```python
from build123d import *

# Parameters (mm, degrees)
BOSS_EXTRUDE1_DEPTH = 31
SKETCH4_W           = 25
SKETCH4_H           = 15
CUT_EXTRUDE2_DEPTH  = 25
CUT_EXTRUDE4_DEPTH  = 11.5
SKETCH7_W           = 31
SKETCH7_H           = 1.7
BOSS_EXTRUDE3_DEPTH = 7
BOSS_EXTRUDE4_DEPTH = 7
LPATTERN1_COUNT     = 8
LPATTERN1_PITCH     = 4
SKETCH11_W          = 12
SKETCH11_H          = 6.5
BOSS_EXTRUDE5_DEPTH = 5.5
FILLET5_R           = 3
SKETCH12_W          = 12
SKETCH12_H          = 6.5
BOSS_EXTRUDE6_DEPTH = 6
CUT_EXTRUDE5_DEPTH  = 12
FILLET6_R           = 2


with BuildPart() as part:
    # Sketch1 → Boss-Extrude1 (new body)
    with BuildSketch(Plane.XY):
        Polygon((0, 0), (0, -30), (12, -30), (12, -20), (5, 0), align=None)
    extrude(amount=-BOSS_EXTRUDE1_DEPTH)

    # Sketch4 → Cut-Extrude2 (cut)
    with BuildSketch(Plane.ZY):
        with Locations((-15, -24.143402944)):
            Rectangle(SKETCH4_W, SKETCH4_H)
    extrude(amount=-CUT_EXTRUDE2_DEPTH, mode=Mode.SUBTRACT)

    # Sketch6 → Cut-Extrude4 (cut, symmetric)
    with BuildSketch(Plane.XY.offset(-15.25)):
        Polygon((5, 0), (5, -14), (9.9, -14), align=None)
    extrude(amount=CUT_EXTRUDE4_DEPTH, both=True, mode=Mode.SUBTRACT)

    # Sketch7 → Boss-Extrude3 (add)
    with BuildSketch(Plane(origin=(0, -25.5, 0), x_dir=(1, 0, 0), z_dir=(0, 1, 0))):
        with Locations((-4.2231607, 26.8)):
            Rectangle(SKETCH7_W, SKETCH7_H)
    extrude(amount=BOSS_EXTRUDE3_DEPTH)

    # Sketch10 → Boss-Extrude4 (add)
    with BuildSketch(Plane(origin=(0, -25.5, 0), x_dir=(1, 0, 0), z_dir=(0, 1, 0))):
        with BuildLine():
            Line((10.353586314, 22.126900466), (9.550714712, 22.126900466))
            ThreePointArc((9.550714712, 22.126900466), (8.911730102, 23.551984668), (9.029666421, 25.109308443))
            ThreePointArc((9.029666421, 25.109308443), (8.752067329, 25.53731984), (8.452150513, 25.95))
            Line((8.452150513, 25.95), (11.452150513, 25.95))
            ThreePointArc((11.452150513, 25.95), (11.152233697, 25.53731984), (10.874634605, 25.109308443))
            ThreePointArc((10.874634605, 25.109308443), (10.992570924, 23.551984668), (10.353586314, 22.126900466))
        make_face()
    boss_extrude4 = extrude(amount=BOSS_EXTRUDE4_DEPTH)

    # LPattern1: Boss-Extrude4 ×8
    with Locations(*[(-i * LPATTERN1_PITCH, 0, 0) for i in range(1, LPATTERN1_COUNT)]):
        add(boss_extrude4)

    # Sketch11 → Boss-Extrude5 (add)
    with BuildSketch(Plane(origin=(0, 0, -31), x_dir=(-1, 0, 0), z_dir=(0, 0, -1))):
        with Locations((-6, -26.75)):
            Rectangle(SKETCH11_W, SKETCH11_H)
    extrude(amount=BOSS_EXTRUDE5_DEPTH)

    # Fillet5
    # the kernel refuses this fillet: 3 mm, written as the material it adds along each edge
    with BuildSketch(Plane(origin=(5, -14, -34.25), x_dir=(0, 1, 0), z_dir=(0, 0, 1))) as fillet5_piece_1_section:
        with BuildLine():
            CenterArc((FILLET5_R, -FILLET5_R), FILLET5_R, 90, 90)
            Line((0, -FILLET5_R), (0, 0))
            Line((0, 0), (FILLET5_R, 0))
        make_face()
    fillet5_piece_1 = extrude(amount=38, mode=Mode.PRIVATE)
    fillet5_piece_1 = split(fillet5_piece_1, bisect_by=Plane(origin=(5.670103817, -13.329896183, -31), z_dir=(0, 0, 1)), keep=Keep.TOP, mode=Mode.PRIVATE)
    fillet5_piece_1 = split(fillet5_piece_1, bisect_by=Plane(origin=(5.670103817, -13.329896183, 0), z_dir=(0, 0, -1)), keep=Keep.TOP, mode=Mode.PRIVATE)
    add(fillet5_piece_1)
    with BuildSketch(Plane(origin=(0, -16.643402944, -2.5), x_dir=(0, -1, 0), z_dir=(1, 0, 0))) as fillet5_piece_2_section:
        with BuildLine():
            CenterArc((FILLET5_R, FILLET5_R), FILLET5_R, 180, 90)
            Line((0, FILLET5_R), (0, 0))
            Line((0, 0), (FILLET5_R, 0))
        make_face()
    fillet5_piece_2 = extrude(amount=18.32519103, mode=Mode.PRIVATE)
    fillet5_piece_2 = split(fillet5_piece_2, bisect_by=Plane(origin=(10.459559167, -15.598740478, -3.164212855), z_dir=(-0.9438583563660173, -0.33035042472810633, 0)), keep=Keep.TOP, mode=Mode.PRIVATE)
    add(fillet5_piece_2)
    with BuildSketch(Plane(origin=(0, -16.643402944, -27.5), x_dir=(0, 0, 1), z_dir=(1, 0, 0))) as fillet5_piece_3_section:
        with BuildLine():
            CenterArc((FILLET5_R, FILLET5_R), FILLET5_R, 180, 90)
            Line((0, FILLET5_R), (0, 0))
            Line((0, 0), (FILLET5_R, 0))
        make_face()
    fillet5_piece_3 = extrude(amount=18.32519103, mode=Mode.PRIVATE)
    fillet5_piece_3 = split(fillet5_piece_3, bisect_by=Plane(origin=(10.435387917, -15.529679764, -26.806522223), z_dir=(-0.9438583563660173, -0.33035042472810633, 0)), keep=Keep.TOP, mode=Mode.PRIVATE)
    add(fillet5_piece_3)

    # Sketch12 → Boss-Extrude6 (add)
    with BuildSketch(Plane.XY):
        with Locations((6, -26.75)):
            Rectangle(SKETCH12_W, SKETCH12_H)
    extrude(amount=BOSS_EXTRUDE6_DEPTH)

    # Sketch13 → Cut-Extrude5 (cut)
    with BuildSketch(Plane.ZY):
        Polygon((-34.3, -25.5), (-27.5, -25.5), (-27.5, -32.069121633), (-31.15, -32.069121633), (-31.15, -29), (-34.3, -29), align=None)
        Polygon((1.037837299, -29), (4.187837299, -29), (4.187837299, -25.5), (-2.612162701, -25.5), (-2.612162701, -32.069121633), (1.037837299, -32.069121633), align=None)
    extrude(amount=-CUT_EXTRUDE5_DEPTH, mode=Mode.SUBTRACT)

    # Fillet6
    fillet6_edges = [part.edges().sort_by_distance(p)[0] for p in [
        (6, -23.5, -31),
        (6, -23.5, -36.5),
        (6, -23.5, 0),
        (6, -23.5, 6),
    ]]
    fillet(fillet6_edges, radius=FILLET6_R)


solid = part.part
```
Geometry: final body of the model. Coordinates: model frame, mm. A direction names the side the tool comes from. Round coordinates to 2 decimals unless told otherwise and drop trailing zeros. Order: outer loops, then holes, each group sorted by start corner. A loop starts at its lowest first (then second) coordinate and runs counter-clockwise, first axis right, second up. Notation, with made-up numbers: (74, 28.25) -> (113, 28.25) arc R29 ccw to (113, 51.25) -> close; hole circle Ø10 at (-29.75, 45). An arc over 180 degrees is marked (long way). Write each question's results on one line, items separated by ' | '.
Q1. Pin query (flat end, axial travel): pin 1 Ø0.8 at (x, z) = (5.5, -33.5) entering from +Y; pin 2 Ø8 at (x, z) = (3.5, -21) entering from -Y; pin 3 Ø0.6 at (x, y) = (11.5, -21) entering from +Z. Return the tip coordinate at first contact, or that it passes through.
Response values:
pin 1: y = -23.5 | pin 2: y = -25.5 | pin 3: z = 0
Q2. Section query B-B (y = -11.75). Output: boundary loops of the cut face in (x, z), and give its area (3 significant figures).
Response values:
outline: (0, -31) -> (9.11, -31) -> (9.11, -26.75) -> (5.1, -26.75) -> (5.1, -3.75) -> (9.11, -3.75) -> (9.11, 0) -> (0, 0) -> close | area: 190 mm²
Q3. Section query C-C (z = -7). Output: boundary loops of the cut face in (x, y), and give its area (3 significant figures).
Response values:
outline: (0, -16.64) -> (10.83, -16.64) -> (9.9, -14) -> (8, -14) arc R3 cw to (5, -11) -> (5, 0) -> (0, 0) -> close | area: 99.3 mm²
Q4. Ray query, line 1 along Z through (x, y) = (5, -27.5); line 2 along Y through (x, z) = (4, -29.5); line 3 along Y through (x, z) = (-14.5, -24.5). Return the intervals inside material, ascending.
Response values:
line 1: -36.5 to -34.3, 4.19 to 6 | line 2: -25.5 to 0 | line 3: -25.5 to -18.5
Q5. Pull-direction query (Y, two-part tool) for faces 5 (the face through (3, 0, -15)), 6 (the face through (5, -13, -31)), 7 (the face through (6, -27, 4.188)), 8 (the face through (6, -27, -34.3)); classes: released by +Y, released by -Y, zero draft, split by the parting line, or undercut.
Response values:
face 5: released by +Y | face 6: zero draft | face 7: undercut | face 8: undercut
Q6. Access query for faces 1 (the face through (4.916, -22.049, -23.53)), 2 (the face through (11.277, -22, -27)), 3 (the face through (-8, -22, -25.95)), 4 (the face through (-1, -25.5, -27)). Directions: +Z, -Z, +X, -X, +Y, -Y. A direction counts if a zero-diameter tool reaches every point of the face in a straight line with its end or side. Return the directions, or none.
Response values:
face 1: -Y | face 2: +X, -Y | face 3: +Z, +Y, -Y | face 4: +X, -X
Q7. Section query A-A (z = -29). Output: boundary loops of the cut face in (x, y).
Response values:
outline: (0, -25.5) -> (12, -25.5) -> (12, -20) -> (5, 0) -> (0, 0) -> close
Q8. Section query D-D (y = -7.5). Output: boundary loops of the cut face in (x, z) (3 decimals).
Response values:
outline: (0, -31) -> (7.625, -31) -> (7.625, -26.75) -> (5, -26.75) -> (5, -3.75) -> (7.625, -3.75) -> (7.625, 0) -> (0, 0) -> close
